Autodesk Inventor part; units mm, degrees
ref_plane "YZ Plane" through (0, 0, 0) normal (1, 0, 0) x (0, 1, 0)
ref_plane "XZ Plane" through (0, 0, 0) normal (0, 1, 0) x (-1, 0, 0)
ref_plane "XY Plane" through (0, 0, 0) normal (0, 0, 1) x (1, 0, 0)
sketch "Sketch1" plane through (0, 0, 0) normal (0, 0, 1) x (1, 0, 0)
  line L0 (0, 0) -> (76.2, 0)
  line L1 (76.2, 0) -> (76.2, 79.0194)
  line L2 (76.2, 79.0194) -> (0, 79.0194)
  line L3 (0, 79.0194) -> (0, 0)
  line L4 (0, 7.3406) -> (-3.175, 7.3406)
  line L5 (-3.175, 7.3406) -> (-3.175, 58.1406)
  line L6 (-3.175, 58.1406) -> (0, 58.1406)
  line L7 (0, 58.1406) -> (0, 7.3406)
  line L8 (38.1, 79.0194) -> (38.1, 15.1376) construction
  line L9 (76.2, 0) -> (0, 0)
  line L10 (76.2, 79.0194) -> (76.2, 0)
  line L11 (76.2, 7.3406) -> (79.375, 7.3406)
  line L12 (79.375, 7.3406) -> (79.375, 58.1406)
  line L13 (79.375, 58.1406) -> (76.2, 58.1406)
  line L14 (76.2, 58.1406) -> (76.2, 7.3406)
  dimension "d0" = 76.2
  dimension "d1" = 79.0194
  dimension "d2" = 7.3406
  dimension "d3" = 50.8
  dimension "d6" = 3.175
extrude "Extrusion1" add sketch "Sketch1" along normal blind 3.175
sketch "Sketch2" plane through (0, 0, 3.175) normal (0, 0, 1) x (1, 0, 0)
  line L0 (76.2, 79.0194) -> (0, 79.0194)
  line L1 (0, 79.0194) -> (76.2, 79.0194)
  line L2 (76.2, 79.0194) -> (76.2, 104.4194)
  line L3 (76.2, 104.4194) -> (0, 104.4194)
  line L4 (0, 104.4194) -> (0, 79.0194)
  point P0 (0, 0)
  dimension "d7" = 25.4
extrude "Extrusion2" add sketch "Sketch2" against normal blind 3.175
sketch "Sketch3" plane through (0, 0, 3.175) normal (0, 0, 1) x (1, 0, 0)
  line L0 (76.2, 104.4194) -> (0, 104.4194)
  line L1 (19.05, 104.4194) -> (57.15, 104.4194)
  line L2 (57.15, 104.4194) -> (57.15, 101.2444)
  line L3 (57.15, 101.2444) -> (19.05, 101.2444)
  line L4 (19.05, 101.2444) -> (19.05, 104.4194)
  line L5 (0, 104.4194) -> (0, 58.1406)
  point P0 (0, 0)
  dimension "d10" = 3.175
  dimension "d11" = 38.1
  dimension "d12" = 19.05
extrude "Extrusion3" cut sketch "Sketch3" against normal blind 3.175
properties part number "back"
CAD build for the part. Positions are in the model's coordinates, mm. A direction names the side the tool comes from. Round coordinates to 2 decimals unless told otherwise and drop trailing zeros. Order: outer loops, then holes, each group sorted by start corner. A loop starts at its lowest first (then second) coordinate and runs counter-clockwise, first axis right, second up. Notation, with made-up numbers: (5.25, -15) - (63.25, -15) arc R18 ccw to (63.25, 0) - close; hole circle Ø11 at (25, 17). An arc over 180 degrees is marked (long way). Answer in a Markdown table with one row per item. Add a question column.
(1) Mould opens along X. For faces 1 (the face through (19.05, 103, 2)), 2 (the face through (-2, 7.341, 2)), 3 (the face through (76.2, 4, 2)), 4 (the face through (0, 82, 2)) say: +X half, -X half, draft (parallel to the pull), parting line (faces both ways), or undercut.
(2) Probe L1, parallel to X at y = 66.5, z = 2.9; L2, parallel to Y at x = 29, z = 1.1. List the from-to ranges inside material, lowest first. Write a range as [from, to].
(3) Drop flat-ended pins along their axis: pin 1 Ø1 at (y, z) = (4, 1.5) entering from +X; pin 2 Ø1 at (x, z) = (54.5, 2) entering from +Y; pin 3 Ø1 at (x, z) = (-1.5, 1) entering from +Y. Give the stop position or say it passes through.
(4) 3-axis set-ups, long thin cutter, end or side, ignore diameter. For faces 5 (the face through (78, 7.341, 2)), 6 (the face through (0, 4, 2)), 7 (the face through (38, 101.244, 2)), 8 (the face through (-2, 58.141, 2)), 9 (the face through (78, 58.141, 2)): which of +Z, -Z, +X, -X, +Y, -Y reach the whole face in a straight line?
(5) Band-saw the part on A-A on z = 1. List the corners of the cut face in (x, y) (3 decimals).
(6) Band-saw the part on B-B on x = 56. List the corners of the cut face in (y, z) (3 decimals), and give its area (3 significant figures).
Data:
| question | item | result |
|---|---|---|
| 1 | face 1 | undercut |
| 1 | face 2 | draft |
| 1 | face 3 | +X half |
| 1 | face 4 | -X half |
| 2 | L1 | x = [0, 76.2] |
| 2 | L2 | y = [0, 101.24] |
| 3 | pin 1 | stops at x = 76.2 |
| 3 | pin 2 | stops at y = 101.24 |
| 3 | pin 3 | stops at y = 58.14 |
| 4 | face 5 | +Z, -Z, +X, -Y |
| 4 | face 6 | +Z, -Z, -X, -Y |
| 4 | face 7 | +Z, -Z, +Y |
| 4 | face 8 | +Z, -Z, -X, +Y |
| 4 | face 9 | +Z, -Z, +X, +Y |
| 5 | outline | (-3.175, 7.341) - (0, 7.341) - (0, 0) - (76.2, 0) - (76.2, 7.341) - (79.375, 7.341) - (79.375, 58.141) - (76.2, 58.141) - (76.2, 104.419) - (57.15, 104.419) - (57.15, 101.244) - (19.05, 101.244) - (19.05, 104.419) - (0, 104.419) - (0, 58.141) - (-3.175, 58.141) - close |
| 6 | outline | (0, 0) - (101.244, 0) - (101.244, 3.175) - (0, 3.175) - close |
| 6 | area | 321 mm^2 |
